Here's how the part is built. I have some questions about the finished solid (model axes, mm). Round coordinates to 2 decimals unless told otherwise and drop trailing zeros. Loops run counter-clockwise (first coordinate to the right, second up) from the corner with the lowest first, then second, coordinate; pieces in that order, holes last. Notation, with made-up numbers: (38.5, 54) - (57.5, 54) arc R5 ccw to (57.5, 59) - close; hole circle Ø3 at (1, 37.25). An arc over 180 degrees is marked (long way). Return JSON: item names as keys, results as strings. Group by question number.
```python
from build123d import *

# Parameters (mm, degrees)
SKETCH1_R           = 1.4
BOSS_EXTRUDE1_DEPTH = 3


with BuildPart() as part:
    # Sketch1 → Boss-Extrude1 (new body)
    with BuildSketch(Plane(origin=(0, 0, 0), x_dir=(1, 0, 0), z_dir=(0, 1, 0))):
        with BuildLine():
            Line((8.498085152, -4.818460921), (8.285834919, 5.179286318))
            ThreePointArc((8.285834919, 5.179286318), (4.712335804, 8.604210269), (1.287411852, 5.030711154))
            ThreePointArc((1.287411852, 5.030711154), (-0.518410861, 0.395144164), (-5.073161201, -1.605787202))
            ThreePointArc((-5.073161201, -1.605787202), (-8.498085152, -5.179286318), (-4.924586037, -8.604210269))
            Line((-4.924586037, -8.604210269), (5.073161201, -8.391960036))
            ThreePointArc((5.073161201, -8.391960036), (7.525719076, -7.314535454), (8.498085152, -4.818460921))
        make_face()
        with Locations((4.786623386, 5.104998736)):
            Circle(SKETCH1_R, mode=Mode.SUBTRACT)
        with Locations((4.998873619, -4.892748502)):
            Circle(SKETCH1_R, mode=Mode.SUBTRACT)
        with Locations((-4.998873619, -5.104998736)):
            Circle(SKETCH1_R, mode=Mode.SUBTRACT)
    extrude(amount=BOSS_EXTRUDE1_DEPTH)


solid = part.part
```
Q1. Please list where these lines run through material, in increasing order: line 1 (Z direction, x = 3.75, y = 2.45); line 2 (X direction, y = 0.25, z = 4); line 3 (Z direction, x = 6, y = 2.85).
Q2. If we mould it in two halves opening along Z, with no side actions, what happens to faces 1 (the cylindrical face through (4.604, 1.479, -6.493)), 2 (the cylindrical face through (-8.5, 1.5, 5.1)), 3 (the flat face through (2, 3, 2))? For each: +Z half, -Z half, draft (parallel to the pull), parting line (faces both ways), or undercut.
Q3. Imagine slicing it at D-D, the plane x = 4.75. List the corners of the cut face in (y, z) for me, and give its area (3 significant figures).
Q4. Imagine slicing it at C-C, the plane y = 2.6. List the corners of the cut face in (x, z) for me (3 decimals), and give its area (3 significant figures).
Q5. Will these pins go through, and if not, where does the flat tip stop? pin 1 Ø1.5 at (x, y) = (-5.5, 0.5) entering from -Z; pin 2 Ø1 at (y, z) = (2, -2) entering from +X.
Q6. Imagine slicing it at A-A, the plane x = -5.5. List the corners of the cut face in (y, z) for me, and give its area (3 significant figures).
Q7. Imagine slicing it at B-B, the plane z = -6.25. List the corners of the cut face in (x, y) for me, and give its area (3 significant figures).
Output values:
{
 "1": {"line 1": "z = -8.45 to -6.05, -4.16 to 4.26, 5.53 to 8.42", "line 2": "x = -8.32 to -5.86, -4.14 to 3.92, 6.08 to 8.48", "line 3": "z = -8.39 to -5.8, -4.41 to 3.91, 5.87 to 8.25"},
 "2": {"face 1": "undercut", "face 2": "parting line", "face 3": "draft"},
 "3": {"outline": "(0, -8.6) - (3, -8.6) - (3, -6.5) - (0, -6.5) - close; (0, -3.71) - (3, -3.71) - (3, 3.52) - (0, 3.52) - close; (0, 6.27) - (3, 6.27) - (3, 8.4) - (0, 8.4) - close", "area": "34.3 mm^2"},
 "4": {"outline": "(-5.073, 1.606) arc R6.5 cw to (1.287, -5.031) arc R3.5 ccw to (8.286, -5.179) - (8.498, 4.818) arc R3.5 ccw to (5.073, 8.392) - (-4.925, 8.604) arc R3.5 ccw to start; hole circle Ø2.8 at (-4.999, 5.105); hole circle Ø2.8 at (4.787, -5.105); hole circle Ø2.8 at (4.999, 4.893)", "area": "166 mm^2"},
 "5": {"pin 1": "stops at z = 1.59", "pin 2": "stops at x = 8.36"},
 "6": {"outline": "(0, 1.64) - (3, 1.64) - (3, 3.8) - (0, 3.8) - close; (0, 6.41) - (3, 6.41) - (3, 8.57) - (0, 8.57) - close", "area": "12.9 mm^2"},
 "7": {"outline": "(1.48, 0) - (3.98, 0) - (3.98, 3) - (1.48, 3) - close; (5.59, 0) - (8.09, 0) - (8.09, 3) - (5.59, 3) - close", "area": "15.0 mm^2"}
}
